Build history of the part. All positions in model axes, mm. A direction names the side the tool comes from. Coordinates: 2 decimals unless noted, no trailing zeros. Loops run counter-clockwise (first coordinate to the right, second up) from the corner with the lowest first, then second, coordinate; pieces in that order, holes last.
(1) Wall check: L1, parallel to X at y = 2, z = -0.65; L2, parallel to X at y = -9, z = -1; L3, parallel to X at y = 9, z = -0.7. Give the ranges that are in metal, low to high.
(2) Slice it at C-C (y = -4). Give the cut face in (x, z).
(3) Tool access for faces 5 (the face through (18.34, -54.43, -0.02)), 6 (the face through (-11.056, -50, 0)), 7 (the face through (11, 1.001, 0)): list every direction of +Z, -Z, +X, -X, +Y, -Y with a clear straight run to the whole face (end or side of a thin tool).
(4) Two-plate mould, pull along X, no slides. Class faces 1 (the face through (-1, -20, 1.5)), 2 (the face through (7.343, 15.431, -0.021)), 3 (the face through (12.16, -44.37, 0.02)), 4 (the face through (-14.056, -15, 0)): pulls with the +X half, pulls with the -X half, needs draft (parallel to the pull), parting line crosses it, or undercut.
(5) Slice it at A-A (z = 0.3). Give the cut face in (x, y).
(6) Slice it at B-B (x = 9). Give the cut face in (y, z).
(7) Flat gauge pins, fed straight in: P1, Ø0.5, axis at x = 16.5, z = -0.5, coming from the +Y side; P2, Ø0.9, axis at y = 9.5, z = -0.5, coming from the +X side; P3, Ø0.9, axis at y = -27.5, z = 0.5, coming from the +X side. Where does each tip first touch, or does it go through?
from build123d import *

# Parameters (mm, degrees)
SKETCH1_W            = 30
SKETCH1_H            = 71
BOSS_EXTRUDE1_DEPTH  = 1.5
SKETCH3_W            = 8
SKETCH3_H            = 15
CUT_EXTRUDE1_DEPTH   = 58.341547982
SKETCH6_W            = 3
SKETCH6_H            = 16
BOSS_EXTRUDE2_DEPTH  = 3
M4_CLEARANCE_HOLE1_D = 4.5
SKETCH9_W            = 3
SKETCH9_H            = 9
CUT_EXTRUDE2_DEPTH   = 59.247041392
FILLET1_R            = 2


with BuildPart() as part:
    # Sketch1 → Boss-Extrude1 (new, symmetric)
    with BuildSketch(Plane.XY):
        with Locations((0.944117647, -19.498529412)):
            Rectangle(SKETCH1_W, SKETCH1_H)
    extrude(amount=BOSS_EXTRUDE1_DEPTH, both=True)

    # Sketch3 → Cut-Extrude1 (cut, through all)
    with BuildSketch(Plane.XY.offset(1.5)):
        with Locations((11.944117647, 8.501470588)):
            Rectangle(SKETCH3_W, SKETCH3_H)
    extrude(amount=-CUT_EXTRUDE1_DEPTH, mode=Mode.SUBTRACT)

    # Sketch6 → Boss-Extrude2 (add)
    with BuildSketch(Plane(origin=(15.944117647, 0, 0), x_dir=(0, 0, -1), z_dir=(1, 0, 0))):
        with Locations((0, -46.998529412)):
            Rectangle(SKETCH6_W, SKETCH6_H)
    extrude(amount=BOSS_EXTRUDE2_DEPTH)

    # M4 Clearance Hole1 (through all)
    with Locations(Plane(origin=(0, 0, -1.5), x_dir=(-1, 0, 0), z_dir=(0, 0, -1))):
        with Locations((7.805882353, 11.001470588), (-13.944117647, -42.998529412)):
            Hole(M4_CLEARANCE_HOLE1_D / 2)

    # Sketch9 → Cut-Extrude2 (cut, through all)
    with BuildSketch(Plane(origin=(0, 0, -1.5), x_dir=(-1, 0, 0), z_dir=(0, 0, -1))):
        with Locations((12.555882353, -50.498529412)):
            Rectangle(SKETCH9_W, SKETCH9_H)
    extrude(amount=-CUT_EXTRUDE2_DEPTH, mode=Mode.SUBTRACT)

    # Fillet1
    fillet1_edges = [part.edges().sort_by_distance(p)[0] for p in [
        (15.944117647, 1.001470588, 0),
        (7.944117647, 16.001470588, 0),
        (18.944117647, -38.998529412, 0),
        (18.944117647, -54.998529412, 0),
        (-14.055882353, -45.998529412, 0),
        (-11.055882353, -54.998529412, 0),
        (-14.055882353, 16.001470588, 0),
    ]]
    fillet(fillet1_edges, radius=FILLET1_R)


solid = part.part
Response values:
1. L1: x = -14.06 to 7.94
1. L2: x = -14.06 to 15.94
1. L3: x = -14.06 to -8.83, -6.78 to 7.94
2. outline: (-14.06, -1.5) - (15.94, -1.5) - (15.94, 1.5) - (-14.06, 1.5) - close
3. face 5: +Z, -Z, +X, -Y
3. face 6: +Z, -Z, -X, -Y
3. face 7: +Z, -Z, +X, +Y
4. face 1: needs draft
4. face 2: pulls with the +X half
4. face 3: undercut
4. face 4: pulls with the -X half
5. outline: (-14.06, -44) arc R2 ccw to (-12.06, -46) - (-11.06, -46) - (-11.06, -53) arc R2 ccw to (-9.06, -55) - (16.94, -55) arc R2 ccw to (18.94, -53) - (18.94, -41) arc R2 ccw to (16.94, -39) - (15.94, -39) - (15.94, -1) arc R2 ccw to (13.94, 1) - (7.94, 1) - (7.94, 14) arc R2 ccw to (5.94, 16) - (-12.06, 16) arc R2 ccw to (-14.06, 14) - close; hole circle Ø4.5 at (-7.81, 11); hole circle Ø4.5 at (13.94, -43)
6. outline: (-55, -1.5) - (1, -1.5) - (1, 1.5) - (-55, 1.5) - close
7. P1: stops at y = -39
7. P2: stops at x = 7.94
7. P3: stops at x = 15.94
